```python
from build123d import *

# Parameters (mm, degrees)
SKETCH1_W           = 12.2
SKETCH1_H           = 13
BOSS_EXTRUDE1_DEPTH = 2
SKETCH1_5_W         = 40
SKETCH1_5_H         = 20
SKETCH1_5_W_2       = 12.2
SKETCH1_5_H_2       = 13
BOSS_EXTRUDE4_DEPTH = 6
SKETCH5_W           = 12.2
SKETCH5_H           = 0.5
CUT_EXTRUDE4_DEPTH  = 2


with BuildPart() as part:
    # Sketch1 → Boss-Extrude1 (new body)
    with BuildSketch(Plane(origin=(0, 0, 0), x_dir=(0, 0, -1), z_dir=(1, 0, 0))):
        with Locations((6.1, 6.5)):
            Rectangle(SKETCH1_W, SKETCH1_H)
    extrude(amount=BOSS_EXTRUDE1_DEPTH)

    # Sketch1<5> → Boss-Extrude4 (add)
    with BuildSketch(Plane(origin=(0, 0, 0), x_dir=(0, 0, -1), z_dir=(1, 0, 0))):
        with Locations((6.1, 6.5)):
            Rectangle(SKETCH1_5_W, SKETCH1_5_H)
        with Locations((6.1, 6.5)):
            Rectangle(SKETCH1_5_W_2, SKETCH1_5_H_2, mode=Mode.SUBTRACT)
    extrude(amount=BOSS_EXTRUDE4_DEPTH)

    # Sketch5 → Cut-Extrude4 (cut)
    with BuildSketch(Plane(origin=(2, 0, 0), x_dir=(0, 0, -1), z_dir=(1, 0, 0))):
        with Locations((6.1, 0.25)):
            Rectangle(SKETCH5_W, SKETCH5_H)
        with Locations((6.1, 12.75)):
            Rectangle(SKETCH5_W, SKETCH5_H)
    extrude(amount=-CUT_EXTRUDE4_DEPTH, mode=Mode.SUBTRACT)


solid = part.part
```
CAD build for the part. Positions are in the model's coordinates, mm. A direction names the side the tool comes from. Round coordinates to 2 decimals unless told otherwise and drop trailing zeros. Order: outer loops, then holes, each group sorted by start corner. A loop starts at its lowest first (then second) coordinate and runs counter-clockwise, first axis right, second up.
Q1. Which spindle directions (+Z, -Z, +X, -X, +Y, -Y) get a long thin tool onto all of the face, cutting with end or side? Do faces 1 (the flat face through (0, 7, -6)), 2 (the flat face through (3, 13, -6)), 3 (the flat face through (4, 6, 0)). Say none if no direction does.
Q2. Slice it at D-D (x = 2.9). Write the cut outline in (y, z), and give its area (3 significant figures).
Q3. Wall check: L1, parallel to Y at x = 1.8, z = -5.5; L2, parallel to Y at x = 5.6, z = -6.5; L3, parallel to Z at x = 2.3, y = 6.75. Give the ranges that are in metal, low to high.
Q4. Slice it at C-C (y = 5.5). Write the cut outline in (x, z).
Q5. Slice it at A-A (z = -10.5). Write the cut outline in (x, y), and give its area (3 significant figures).
Q6. Two-plate mould, pull along Y, no slides. Class faces 4 (the flat face through (1, 0.5, -6)), 5 (the flat face through (4, 6, -12.2)), 6 (the flat face through (6, 13.3, -5.8)), 7 (the flat face through (3, 16.5, -6)): pulls with the +Y half, pulls with the -Y half, needs draft (parallel to the pull), parting line crosses it, or undercut.
Q7. Slice it at B-B (x = 1.3). Write the cut outline in (y, z), and give its area (3 significant figures).
Results below:
1. face 1: +Z, -Z, -X, +Y, -Y
1. face 2: +X, -X
1. face 3: +X
2. outline: (-3.5, -26.1) - (16.5, -26.1) - (16.5, 13.9) - (-3.5, 13.9) - close; hole (0, -12.2) - (13, -12.2) - (13, 0) - (0, 0) - close
2. area: 641 mm2
3. L1: y = -3.5 to 0, 0.5 to 12.5, 13 to 16.5
3. L2: y = -3.5 to 0, 13 to 16.5
3. L3: z = -26.1 to -12.2, 0 to 13.9
4. outline: (0, -26.1) - (6, -26.1) - (6, -12.2) - (2, -12.2) - (2, 0) - (6, 0) - (6, 13.9) - (0, 13.9) - close
5. outline: (0, -3.5) - (6, -3.5) - (6, 0) - (0, 0) - close; (0, 0.5) - (2, 0.5) - (2, 12.5) - (0, 12.5) - close; (0, 13) - (6, 13) - (6, 16.5) - (0, 16.5) - close
5. area: 66.0 mm2
6. face 4: undercut
6. face 5: undercut
6. face 6: needs draft
6. face 7: pulls with the +Y half
7. outline: (-3.5, -26.1) - (16.5, -26.1) - (16.5, 13.9) - (-3.5, 13.9) - close; hole (0, -12.2) - (0.5, -12.2) - (0.5, 0) - (0, 0) - close; hole (12.5, -12.2) - (13, -12.2) - (13, 0) - (12.5, 0) - close
7. area: 788 mm2
